Source: CAD feature listing. Evaluate the final solid. Frame: model axes, mm. A direction names the side the tool comes from. Give positions to 0.01 mm unless a question says otherwise; leave off trailing zeros. Loops run counter-clockwise (first coordinate to the right, second up) from the corner with the lowest first, then second, coordinate; pieces in that order, holes last.
from build123d import *

# Parameters (mm, degrees)
SKETCH_1_W                 = 153.4
SKETCH_1_H                 = 10
EXTRUDE_1_DEPTH            = 3
CUT_EXTRUDE_1_DEPTH        = 4
PATTERN_LINEAR_1_COUNT     = 21
PATTERN_LINEAR_1_PITCH     = 6.28
PATTERN_LINEAR_1_COL_COUNT = 2
PATTERN_LINEAR_1_COL_PITCH = 6.28
SKETCH_3_W                 = 10
SKETCH_3_H                 = 15
EXTRUDE_2_DEPTH            = 10
FILLET_1_R                 = 5
SKETCH_4_R                 = 1.25
CUT_EXTRUDE_2_DEPTH        = 5.5


with BuildPart() as part:
    # 스케치1 → 보스-돌출1 (new body)
    with BuildSketch(Plane.XY):
        with Locations((0, 5)):
            Rectangle(SKETCH_1_W, SKETCH_1_H)
    extrude(amount=-EXTRUDE_1_DEPTH)

    # 스케치2 → 컷-돌출1 (cut, through all)
    with BuildSketch(Plane.XY):
        Polygon((-68.600074414, 5.5), (-67.279925586, 5.5), (-65.642059531, 10), (-70.237940469, 10), align=None)
    cut_extrude_1 = extrude(amount=-CUT_EXTRUDE_1_DEPTH, mode=Mode.SUBTRACT)

    # 선형 패턴1: 컷-돌출1 ×21
    with Locations(*[(i * PATTERN_LINEAR_1_PITCH, 0, 0) for i in range(1, PATTERN_LINEAR_1_COUNT)]):
        add(cut_extrude_1, mode=Mode.SUBTRACT)

    # 선형 패턴1 col: 컷-돌출1 ×2
    with Locations(*[(-i * PATTERN_LINEAR_1_COL_PITCH, 0, 0) for i in range(1, PATTERN_LINEAR_1_COL_COUNT)]):
        add(cut_extrude_1, mode=Mode.SUBTRACT)

    # 스케치3 → 보스-돌출2 (add)
    with BuildSketch(Plane.XZ):
        with Locations((71.7, 4.5)):
            Rectangle(SKETCH_3_W, SKETCH_3_H)
    extrude(amount=-EXTRUDE_2_DEPTH)

    # 필렛1
    fillet_1_edges = [part.edges().sort_by_distance(p)[0] for p in [
        (66.7, 5, 0),
    ]]
    fillet(fillet_1_edges, radius=FILLET_1_R)

    # 스케치4 → 컷-돌출2 (cut)
    with BuildSketch(Plane.XZ):
        with Locations((71.7, 9)):
            Circle(SKETCH_4_R)
    extrude(amount=-CUT_EXTRUDE_2_DEPTH, mode=Mode.SUBTRACT)


solid = part.part
1) Ray query, probe 1 along Z at (x, y) = (71.7, 1.9); probe 2 along Z at (x, y) = (-41, 3); probe 3 along X at (y, z) = (3, 4.5). Return the intervals inside material, ascending.
Checks:
probe 1: z = -3 to 7.75, 10.25 to 12
probe 2: z = -3 to 0
probe 3: x = 66.67 to 76.7
2) Cut plane B-B (x = 71.7). Return loops of the section in (y, z).
Checks:
outline: (0, -3) - (10, -3) - (10, 12) - (0, 12) - (0, 10.25) - (5.5, 10.25) - (5.5, 7.75) - (0, 7.75) - close
3) Cut plane C-C (y = 7.25). State how many separate pieces and enclosed holes the cut face has, and give its area (3 significant figures).
Checks:
separate pieces: 23
enclosed holes: 0
area: 414 mm2
4) Contact query for flat-ended pins moving along their axis: P1, Ø1.5, axis at x = 9, y = 9, coming from the -Z side; P2, Ø0.7, axis at x = 45, z = -2, coming from the +Y side; P3, Ø0.8, axis at x = 72, z = 9.5, coming from the -Y side. Output: stop coordinate, or through.
Checks:
P1: stops at z = -3
P2: stops at y = 5.5
P3: stops at y = 5.5
5) Cut plane A-A (z = 9). Return loops of the section in (x, y), and give its area (4 significant figures).
Checks:
outline: (66.7, 0) - (70.45, 0) - (70.45, 5.5) - (72.95, 5.5) - (72.95, 0) - (76.7, 0) - (76.7, 10) - (66.7, 10) - close
area: 86.25 mm2
6) Reachability of faces 1 (the flat face through (70, 10, 3)), 2 (the flat face through (-9.95, 7.72, -1.48)) from +Z, -Z, +X, -X, +Y, -Y: full face, straight path, thin tool, end or side. Return the list, or none.
Checks:
face 1: +Z, -Z, +X, -X, +Y
face 2: +Z, -Z, +Y
